from build123d import *

# Parameters (mm, degrees)
SKETCH3_R                = 9.525
SKETCH3_R_2              = 2.38125
BOSS_EXTRUDE1_DEPTH      = 6.35
BOSS_EXTRUDE1_DEPTH_BACK = 7.9375
SKETCH4_R                = 4.7625
CUT_EXTRUDE1_DEPTH       = 6.35
SKETCH5_W                = 4.1275
SKETCH5_H                = 0.0635
FILLET2_R                = 1.651


with BuildPart() as part:
    # Sketch3 → Boss-Extrude1 (new body, two sides)
    with BuildSketch(Plane(origin=(0, 0, 0), x_dir=(1, 0, 0), z_dir=(0, 1, 0))) as boss_extrude1_sk:
        Circle(SKETCH3_R)
        Circle(SKETCH3_R_2, mode=Mode.SUBTRACT)
    extrude(amount=BOSS_EXTRUDE1_DEPTH)
    extrude(boss_extrude1_sk.sketch, amount=-BOSS_EXTRUDE1_DEPTH_BACK)

    # Sketch4 → Cut-Extrude1 (cut)
    with BuildSketch(Plane(origin=(0, 0, 0), x_dir=(1, 0, 0), z_dir=(0, 1, 0))):
        Circle(SKETCH4_R)
    extrude(amount=CUT_EXTRUDE1_DEPTH, mode=Mode.SUBTRACT)

    # Sketch5 → Cut-Revolve1 (revolve, cut)
    with BuildSketch(Plane.XY):
        with Locations((-7.46125, 6.31825)):
            Rectangle(SKETCH5_W, SKETCH5_H)
    revolve(axis=Axis((0, -7.9375, 0), (0, 1, 0)), mode=Mode.SUBTRACT)

    # Fillet2
    fillet2_edges = [part.edges().sort_by_distance(p)[0] for p in [
        (-9.525, 6.2865, 0),
    ]]
    fillet(fillet2_edges, radius=FILLET2_R)


solid = part.part
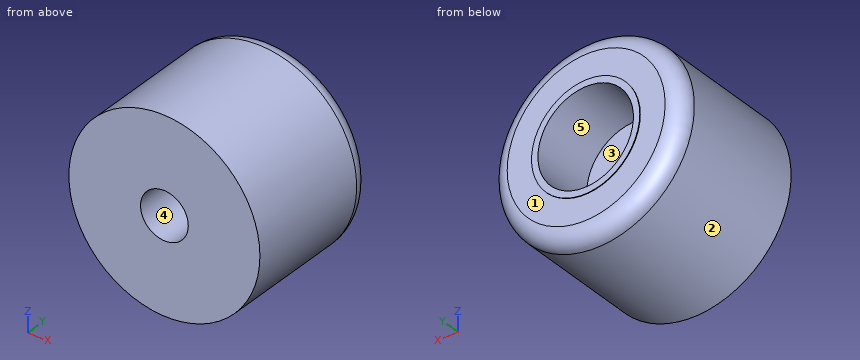
Read the model definition and answer for the solid it produces. Units are mm, in the model's axes. Face numbers are marked on the shaded views. A direction names the side the tool comes from. Give positions to 0.01 mm unless a question says otherwise; leave off trailing zeros. Answer in a Markdown table with one row per item. Add a question column.
Item 1: Flat-ended cylindrical pins translate along their axes: P1, Ø6, axis at x = 0, z = 0, coming from the +Y side; P2, Ø8, axis at y = -1.5, z = -7.5, coming from the -X side; P3, Ø2, axis at x = -6, z = -6, coming from the +Y side. Find the tip coordinate at first contact, or state that the pin passes through.
Item 2: Determine the mould class of the marked faces 1, 2 and 3 for opening direction X: pulls with the +X half, pulls with the -X half, needs draft (parallel to the pull), parting line crosses it, or undercut.
Item 3: A tool of negligible diameter and unlimited length cuts with its end or side. For the marked faces 4 and 5, from which of +Z, -Z, +X, -X, +Y, -Y can it reach the whole face along a straight path? Write none if from no direction.
Item 4: Find the intervals of material crossed by L1, parallel to X at y = 2.75, z = 0 (1 decimal); L2, parallel to X at y = -6, z = 0 (3 decimals), in increasing order.
Recorded:
| question | item | result |
|---|---|---|
| 1 | P1 | stops at y = 0 |
| 1 | P2 | stops at x = -8.86 |
| 1 | P3 | stops at y = 6.29 |
| 2 | face 1 | needs draft |
| 2 | face 2 | parting line crosses it |
| 2 | face 3 | undercut |
| 3 | face 4 | +Y, -Y |
| 3 | face 5 | +Y |
| 4 | L1 | x = -9.5 to -4.8, 4.8 to 9.5 |
| 4 | L2 | x = -9.525 to -2.381, 2.381 to 9.525 |
